Answer from the drawing. Dimensions are ordinates in mm from the lowest x, y and z of the part. Coordinates: 2 decimals unless noted, no trailing zeros. Order: outer loops, then holes, each group sorted by start corner. A loop starts at its lowest first (then second) coordinate and runs counter-clockwise, first axis right, second up.
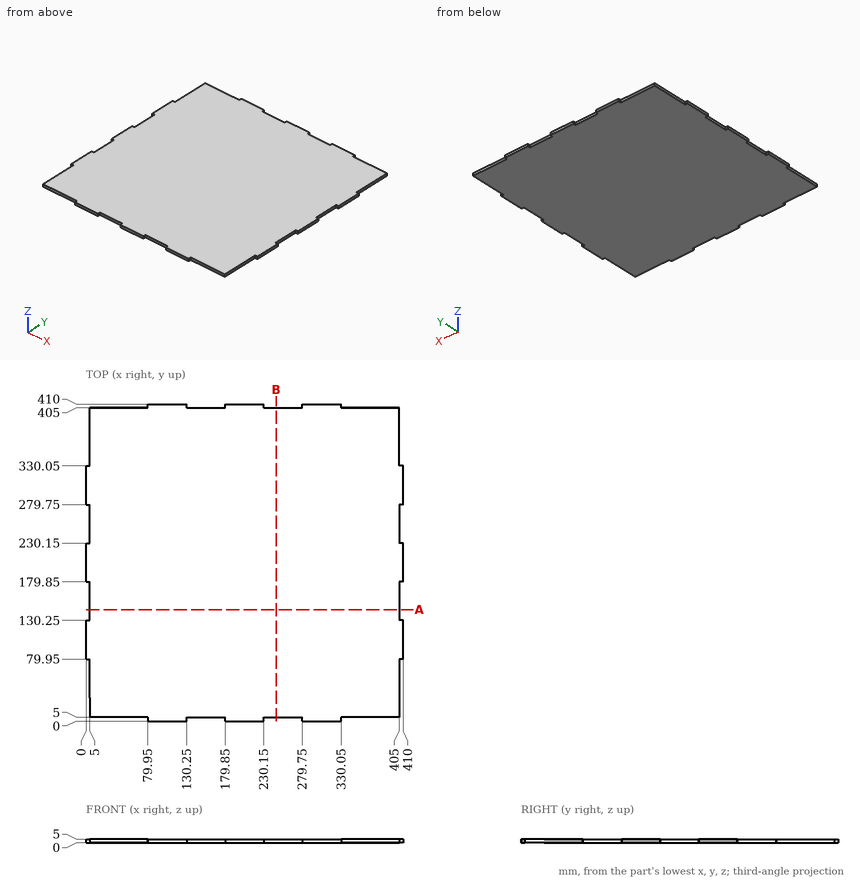
1. Flat-ended cylindrical pins translate along their axes: pin 1 (2.5 mm diameter, centred on y = 407, z = 2.5, fed in from -X); pin 2 (1.5 mm diameter, centred on y = 384, z = 2.5, fed in from +X); pin 3 (1.5 mm diameter, centred on x = 61, z = 3.5, fed in from -Y). Find the tip coordinate at first contact, or state that the pin passes through.
2. Consider probe 1 along X at (y, z) = (20, 0.65). Determine where the line is inside the solid, lowest interval first.
3. The part is cut by section A-A (y = 144). Determine the outline of the cut face in (x, z), plus the area to 3 significant figures.
Worked out:
1. pin 1: stops at x = 79.95
1. pin 2: stops at x = 405
1. pin 3: stops at y = 5
2. probe 1: x = 5 to 405
3. outline: (5, 0) - (405, 0) - (405, 5) - (5, 5) - close
3. area: 2,000 mm2
